Part model, mm, in its own coordinate system. Coordinates: 2 decimals unless noted, no trailing zeros. Loops run counter-clockwise (first coordinate to the right, second up) from the corner with the lowest first, then second, coordinate; pieces in that order, holes last. Notation, with made-up numbers: M 77,48 L 124,48 A19 ccw 124,67 Z; hole C 68,69 d8. An arc over 180 degrees is marked long. Use a Markdown table: item, result. Add a question column.
1) Band-saw the part on A-A (x = 379). List the corners of the cut face in (y, z), plus the area to 3 significant figures.
2) Band-saw the part on B-B (z = 3.5). List the corners of the cut face in (x, y).
3) Wall check: probe 1 along Y at (x, z) = (420, 12.5); probe 2 along X at (y, z) = (661.5, 12.5). Give the ranges that are in metal, low to high. Write a range as from..to.
from build123d import *

# Parameters (mm, degrees)
F0_W     = 508
F0_H     = 355.6
F1_DEPTH = 17.78


with BuildPart() as f1:
    # F0 (on Top) → F1 (new body)
    with BuildSketch(Plane.XY):
        with Locations((254, 177.8)):
            Rectangle(F0_W, F0_H)
        Polygon((177.8, 50.8), (177.8, 33.02), (76.2, 33.02), (76.2, 50.8), (127, 50.8), align=None, mode=Mode.SUBTRACT)
        Polygon((330.2, 33.02), (330.2, 50.8), (381, 50.8), (431.8, 50.8), (431.8, 33.02), align=None, mode=Mode.SUBTRACT)
        Polygon((0, 660.4), (0, 355.6), (508, 355.6), (508, 711.2), (254, 711.2), (0, 711.2), align=None)
        Polygon((177.8, 660.4), (127, 660.4), (76.2, 660.4), (76.2, 678.18), (177.8, 678.18), align=None, mode=Mode.SUBTRACT)
        Polygon((431.8, 660.4), (381, 660.4), (330.2, 660.4), (330.2, 678.18), (431.8, 678.18), align=None, mode=Mode.SUBTRACT)
    extrude(amount=F1_DEPTH)


solid = f1.part
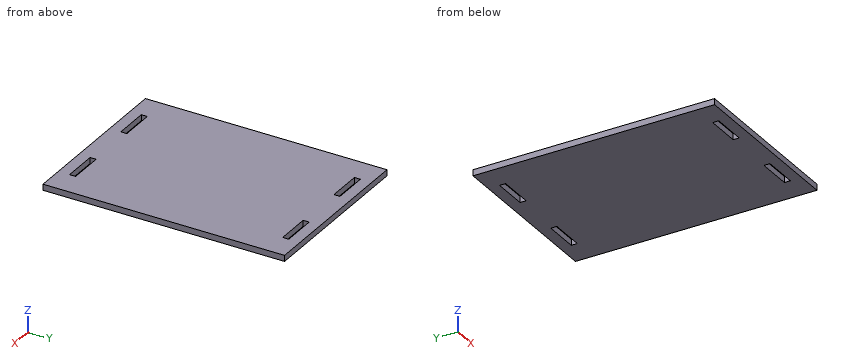
Entries:
| question | item | result |
|---|---|---|
| 1 | outline | M 0,0 L 33.02,0 L 33.02,17.78 L 0,17.78 Z; M 50.8,0 L 660.4,0 L 660.4,17.78 L 50.8,17.78 Z; M 678.18,0 L 711.2,0 L 711.2,17.78 L 678.18,17.78 Z |
| 1 | area | 12,000 mm2 |
| 2 | outline | M 0,0 L 508,0 L 508,711.2 L 0,711.2 Z; hole M 76.2,33.02 L 177.8,33.02 L 177.8,50.8 L 76.2,50.8 Z; hole M 76.2,660.4 L 177.8,660.4 L 177.8,678.18 L 76.2,678.18 Z; hole M 330.2,33.02 L 431.8,33.02 L 431.8,50.8 L 330.2,50.8 Z; hole M 330.2,660.4 L 431.8,660.4 L 431.8,678.18 L 330.2,678.18 Z |
| 3 | probe 1 | 0..33.02, 50.8..660.4, 678.18..711.2 |
| 3 | probe 2 | 0..76.2, 177.8..330.2, 431.8..508 |
